Job drawing, mm, ordinate dimensions from the low corner. One solid piece. Round coordinates to 2 decimals unless told otherwise and drop trailing zeros. Loops run counter-clockwise (first coordinate to the right, second up) from the corner with the lowest first, then second, coordinate; pieces in that order, holes last. Notation, with made-up numbers: M 77.5,15 L 136.5,15 A28 cw 136.5,33 Z; hole C 6.25,-29 d10. An arc over 180 degrees is marked long. One line per item, written item: value.
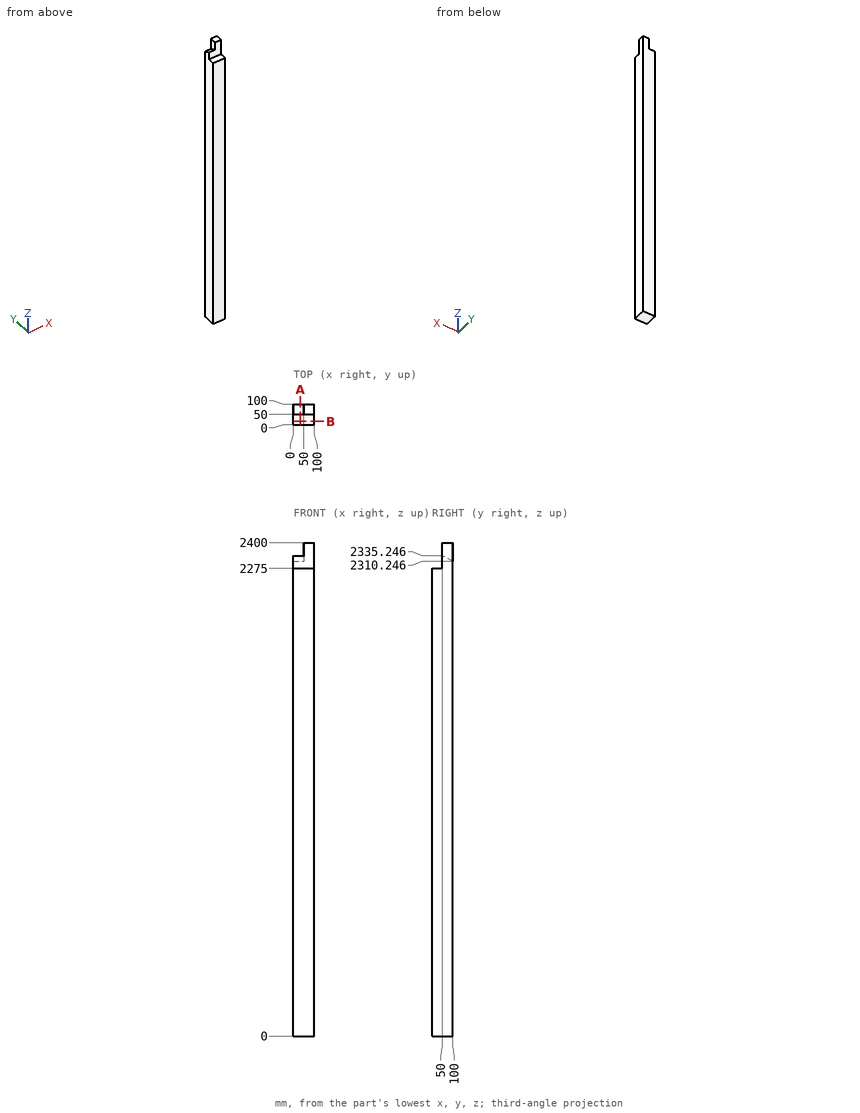
Item 1: Drop flat-ended pins along their axis: P1, Ø2, axis at x = 21.5, y = 61, coming from the -Z side; P2, Ø8, axis at x = 37, y = 33.5, coming from the +Z side. Give the stop position or say it passes through.
Check values:
P1: stops at z = 0
P2: stops at z = 2275
Item 2: Wall check: line 1 along Z through (x, y) = (21, 16.5); line 2 along Z through (x, y) = (10, 90). Give the ranges that are in metal, low to high.
Check values:
line 1: z = 0 to 2275
line 2: z = 0 to 2315.25
Item 3: Slice it at B-B, the plane y = 15.5. Give the cut face in (x, z).
Check values:
outline: M 0,0 L 100,0 L 100,2275 L 0,2275 Z
Item 4: Slice it at A-A, the plane x = 34. Give the cut face in (y, z).
Check values:
outline: M 0,0 L 100,0 L 100,2310.25 L 50,2335.25 L 50,2275 L 0,2275 Z
